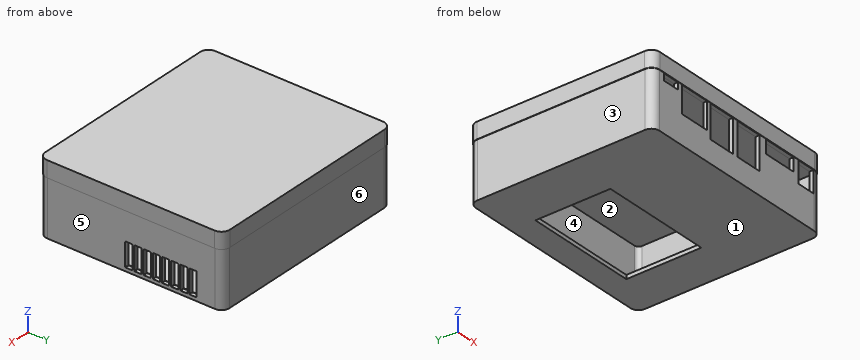
```python
from build123d import *

# Parameters (mm, degrees)
BOSS_EXTRUDE1_DEPTH = 2
BOSS_EXTRUDE2_DEPTH = 8.3
SKETCH3_W           = 57.8
SKETCH3_H           = 38.4
BOSS_EXTRUDE3_DEPTH = 2
BOSS_EXTRUDE6_DEPTH = 30
SKETCH5_W           = 9.3
SKETCH5_H           = 11
SKETCH5_W_2         = 17.696
SKETCH5_H_2         = 6.81
SKETCH5_W_3         = 14.05
SKETCH5_H_3         = 16.84
SKETCH5_W_4         = 8.89
SKETCH5_H_4         = 3.43
SKETCH5_W_5         = 8.74
SKETCH5_H_5         = 13.649992795
SKETCH5_W_6         = 2
SKETCH5_W_7         = 1.707
CUT_EXTRUDE1_DEPTH  = 2
CUT_EXTRUDE2_DEPTH  = 2
CUT_EXTRUDE3_DEPTH  = 2
CUT_EXTRUDE4_DEPTH  = 2


with BuildPart() as part:
    # Sketch1 → Boss-Extrude1 (new body)
    with BuildSketch(Plane.XY):
        with BuildLine():
            Line((-86.3, 47.45), (-86.3, -38.45))
            ThreePointArc((-86.3, -38.45), (-85.626345597, -40.076345597), (-84, -40.75))
            Line((-84, -40.75), (14.4, -40.75))
            ThreePointArc((14.4, -40.75), (16.026345597, -40.076345597), (16.7, -38.45))
            Line((16.7, -38.45), (16.7, 47.45))
            ThreePointArc((16.7, 47.45), (16.026345597, 49.076345597), (14.4, 49.75))
            Line((14.4, 49.75), (-84, 49.75))
            ThreePointArc((-84, 49.75), (-85.626345597, 49.076345597), (-86.3, 47.45))
        make_face()
    extrude(amount=BOSS_EXTRUDE1_DEPTH)

    # Sketch2 → Boss-Extrude2 (add)
    with BuildSketch(Plane.XY.offset(2)):
        with BuildLine():
            Line((-88.3, 47.45), (-88.3, -38.45))
            ThreePointArc((-88.3, -38.45), (-87.040559159, -41.490559159), (-84, -42.75))
            Line((-84, -42.75), (14.4, -42.75))
            ThreePointArc((14.4, -42.75), (17.440559159, -41.490559159), (18.7, -38.45))
            Line((18.7, -38.45), (18.7, 47.45))
            ThreePointArc((18.7, 47.45), (17.440559159, 50.490559159), (14.4, 51.75))
            Line((14.4, 51.75), (-84, 51.75))
            ThreePointArc((-84, 51.75), (-87.040559159, 50.490559159), (-88.3, 47.45))
        make_face()
    extrude(amount=-BOSS_EXTRUDE2_DEPTH)



with BuildPart() as body_2:
    # Sketch3 → Boss-Extrude3 (new body)
    with BuildSketch(Plane(origin=(0, 0, -34.766), x_dir=(-1, 0, 0), z_dir=(0, 0, -1))):
        with BuildLine():
            Line((-14.4, -40.55), (84, -40.55))
            ThreePointArc((84, -40.55), (85.48492424, -39.93492424), (86.1, -38.45))
            Line((86.1, -38.45), (86.1, 47.45))
            ThreePointArc((86.1, 47.45), (85.48492424, 48.93492424), (84, 49.55))
            Line((84, 49.55), (-14.4, 49.55))
            ThreePointArc((-14.4, 49.55), (-15.88492424, 48.93492424), (-16.5, 47.45))
            Line((-16.5, 47.45), (-16.5, -38.45))
            ThreePointArc((-16.5, -38.45), (-15.88492424, -39.93492424), (-14.4, -40.55))
        make_face()
        with Locations((32.8, 19.76)):
            Rectangle(SKETCH3_W, SKETCH3_H, mode=Mode.SUBTRACT)
    extrude(amount=-BOSS_EXTRUDE3_DEPTH)


with BuildPart() as part_1:
    add(part.part)

    add(body_2.part)  # Boss-Extrude6 merges body 2
    # Sketch4 → Boss-Extrude6 (add)
    with BuildSketch(Plane(origin=(0, 0, -34.766), x_dir=(-1, 0, 0), z_dir=(0, 0, -1))):
        with BuildLine():
            Line((84, 51.55), (-14.4, 51.55))
            ThreePointArc((-14.4, 51.55), (-17.299137803, 50.349137803), (-18.5, 47.45))
            Line((-18.5, 47.45), (-18.5, -38.45))
            ThreePointArc((-18.5, -38.45), (-17.299137803, -41.349137803), (-14.4, -42.55))
            Line((-14.4, -42.55), (84, -42.55))
            ThreePointArc((84, -42.55), (86.899137803, -41.349137803), (88.1, -38.45))
            Line((88.1, -38.45), (88.1, 47.45))
            ThreePointArc((88.1, 47.45), (86.899137803, 50.349137803), (84, 51.55))
        make_face()
        with BuildLine():
            ThreePointArc((-16.5, -38.45), (-15.88492424, -39.93492424), (-14.4, -40.55))
            Line((-14.4, -40.55), (84, -40.55))
            ThreePointArc((84, -40.55), (85.48492424, -39.93492424), (86.1, -38.45))
            Line((86.1, -38.45), (86.1, 47.45))
            ThreePointArc((86.1, 47.45), (85.48492424, 48.93492424), (84, 49.55))
            Line((84, 49.55), (-14.4, 49.55))
            ThreePointArc((-14.4, 49.55), (-15.88492424, 48.93492424), (-16.5, 47.45))
            Line((-16.5, 47.45), (-16.5, -38.45))
        make_face(mode=Mode.SUBTRACT)
    extrude(amount=-BOSS_EXTRUDE6_DEPTH)

    # Sketch5 → Cut-Extrude1 (cut)
    with BuildSketch(Plane.XZ.offset(42.55)):
        with Locations((9.2, -11.97)):
            Rectangle(SKETCH5_W, SKETCH5_H)
        with Locations((-7.56, -9.9512)):
            Rectangle(SKETCH5_W_2, SKETCH5_H_2)
        with Locations((-27.4, -14.9662)):
            Rectangle(SKETCH5_W_3, SKETCH5_H_3)
        with Locations((-44.4, -14.9662)):
            Rectangle(SKETCH5_W_3, SKETCH5_H_3)
        with Locations((-76.775, -8.2612)):
            Rectangle(SKETCH5_W_4, SKETCH5_H_4)
        with Locations((-61.75, -13.294996398)):
            Rectangle(SKETCH5_W_5, SKETCH5_H_5)
        with Locations((-56.38, -13.294996398)):
            Rectangle(SKETCH5_W_6, SKETCH5_H_5)
        with Locations((-67.12, -13.294996398)):
            Rectangle(SKETCH5_W_6, SKETCH5_H_5)
        with Locations((-54.5265, -13.294996398)):
            Rectangle(SKETCH5_W_7, SKETCH5_H_5)
        with Locations((-68.9735, -13.294996398)):
            Rectangle(SKETCH5_W_7, SKETCH5_H_5)
    extrude(amount=-CUT_EXTRUDE1_DEPTH, mode=Mode.SUBTRACT)

    # Sketch6 → Cut-Extrude2 (cut)
    with BuildSketch(Plane(origin=(18.5, 0, 0), x_dir=(0, 0, -1), z_dir=(1, 0, 0))):
        with BuildLine():
            Line((32.966, 1.76), (32.966, 4.86))
            ThreePointArc((32.966, 4.86), (32.878132034, 5.072132034), (32.666, 5.16))
            Line((32.666, 5.16), (21.066, 5.16))
            ThreePointArc((21.066, 5.16), (20.853867966, 5.072132034), (20.766, 4.86))
            Line((20.766, 4.86), (20.766, 1.76))
            ThreePointArc((20.766, 1.76), (20.853867966, 1.547867966), (21.066, 1.46))
            Line((21.066, 1.46), (32.666, 1.46))
            ThreePointArc((32.666, 1.46), (32.878132034, 1.547867966), (32.966, 1.76))
        make_face()
    extrude(amount=-CUT_EXTRUDE2_DEPTH, mode=Mode.SUBTRACT)

    # Sketch7 → Cut-Extrude3 (cut)
    with BuildSketch(Plane(origin=(18.5, 0, 0), x_dir=(0, 0, -1), z_dir=(1, 0, 0))):
        with BuildLine():
            Line((20.766, 28.36), (20.766, 25.26))
            ThreePointArc((20.766, 25.26), (20.853867966, 25.047867966), (21.066, 24.96))
            Line((21.066, 24.96), (32.666, 24.96))
            ThreePointArc((32.666, 24.96), (32.878132034, 25.047867966), (32.966, 25.26))
            Line((32.966, 25.26), (32.966, 28.36))
            ThreePointArc((32.966, 28.36), (32.878132034, 28.572132034), (32.666, 28.66))
            Line((32.666, 28.66), (21.066, 28.66))
            ThreePointArc((21.066, 28.66), (20.853867966, 28.572132034), (20.766, 28.36))
        make_face()
        with BuildLine():
            Line((32.666, 23.96), (21.066, 23.96))
            ThreePointArc((21.066, 23.96), (20.853867966, 23.872132034), (20.766, 23.66))
            Line((20.766, 23.66), (20.766, 20.56))
            ThreePointArc((20.766, 20.56), (20.853867966, 20.347867966), (21.066, 20.26))
            Line((21.066, 20.26), (32.666, 20.26))
            ThreePointArc((32.666, 20.26), (32.878132034, 20.347867966), (32.966, 20.56))
            Line((32.966, 20.56), (32.966, 23.66))
            ThreePointArc((32.966, 23.66), (32.878132034, 23.872132034), (32.666, 23.96))
        make_face()
        with BuildLine():
            Line((32.666, 15.56), (21.066, 15.56))
            ThreePointArc((21.066, 15.56), (20.853867966, 15.647867966), (20.766, 15.86))
            Line((20.766, 15.86), (20.766, 18.96))
            ThreePointArc((20.766, 18.96), (20.853867966, 19.172132034), (21.066, 19.26))
            Line((21.066, 19.26), (32.666, 19.26))
            ThreePointArc((32.666, 19.26), (32.878132034, 19.172132034), (32.966, 18.96))
            Line((32.966, 18.96), (32.966, 15.86))
            ThreePointArc((32.966, 15.86), (32.878132034, 15.647867966), (32.666, 15.56))
        make_face()
        with BuildLine():
            Line((32.666, 14.56), (21.066, 14.56))
            ThreePointArc((21.066, 14.56), (20.853867966, 14.472132034), (20.766, 14.26))
            Line((20.766, 14.26), (20.766, 11.16))
            ThreePointArc((20.766, 11.16), (20.853867966, 10.947867966), (21.066, 10.86))
            Line((21.066, 10.86), (32.666, 10.86))
            ThreePointArc((32.666, 10.86), (32.878132034, 10.947867966), (32.966, 11.16))
            Line((32.966, 11.16), (32.966, 14.26))
            ThreePointArc((32.966, 14.26), (32.878132034, 14.472132034), (32.666, 14.56))
        make_face()
        with BuildLine():
            Line((20.766, 9.56), (20.766, 6.46))
            ThreePointArc((20.766, 6.46), (20.853867966, 6.247867966), (21.066, 6.16))
            Line((21.066, 6.16), (32.666, 6.16))
            ThreePointArc((32.666, 6.16), (32.878132034, 6.247867966), (32.966, 6.46))
            Line((32.966, 6.46), (32.966, 9.56))
            ThreePointArc((32.966, 9.56), (32.878132034, 9.772132034), (32.666, 9.86))
            Line((32.666, 9.86), (21.066, 9.86))
            ThreePointArc((21.066, 9.86), (20.853867966, 9.772132034), (20.766, 9.56))
        make_face()
    extrude(amount=-CUT_EXTRUDE3_DEPTH, mode=Mode.SUBTRACT)

    # Sketch10 → Cut-Extrude4 (cut)
    with BuildSketch(Plane(origin=(18.5, 0, 0), x_dir=(0, 0, -1), z_dir=(1, 0, 0))):
        with BuildLine():
            Line((32.966, 34.66), (32.966, 37.76))
            ThreePointArc((32.966, 37.76), (32.878132034, 37.972132034), (32.666, 38.06))
            Line((32.666, 38.06), (21.066, 38.06))
            ThreePointArc((21.066, 38.06), (20.853867966, 37.972132034), (20.766, 37.76))
            Line((20.766, 37.76), (20.766, 34.66))
            ThreePointArc((20.766, 34.66), (20.853867966, 34.447867966), (21.066, 34.36))
            Line((21.066, 34.36), (32.666, 34.36))
            ThreePointArc((32.666, 34.36), (32.878132034, 34.447867966), (32.966, 34.66))
        make_face()
        with BuildLine():
            Line((20.766, 33.06), (20.766, 29.96))
            ThreePointArc((20.766, 29.96), (20.853867966, 29.747867966), (21.066, 29.66))
            Line((21.066, 29.66), (32.666, 29.66))
            ThreePointArc((32.666, 29.66), (32.878132034, 29.747867966), (32.966, 29.96))
            Line((32.966, 29.96), (32.966, 33.06))
            ThreePointArc((32.966, 33.06), (32.878132034, 33.272132034), (32.666, 33.36))
            Line((32.666, 33.36), (21.066, 33.36))
            ThreePointArc((21.066, 33.36), (20.853867966, 33.272132034), (20.766, 33.06))
        make_face()
    extrude(amount=-CUT_EXTRUDE4_DEPTH, mode=Mode.SUBTRACT)


solid = part_1.part
```
Check sheet for the modelled part. Datum: model origin and axes. Units: mm. Face numbers are marked on the shaded views. A direction names the side the tool comes from. Give positions to 0.01 mm unless a question says otherwise; leave off trailing zeros. Write each loop counter-clockwise with the first axis right and the second up, starting at its lowest first coordinate (ties: lowest second). Pieces come first, ordered by that corner, then holes.
Item 1: Cross-section at C-C (z = -15). Count the separate pieces of the cut face and the enclosed holes in it, and give its area (3 significant figures).
Item 2: Cross-section at B-B (y = 12.5). Enter the section's corners in (x, z).
Item 3: Access from +Z, -Z, +X, -X, +Y, -Y to the whole of each face (thin tool, end or side, straight path). Record for the marked faces 4, 5 and 6.
Item 4: Draft check along Z on the marked faces 1, 2 and 3. Enter one of: released by +Z, released by -Z, zero draft, split by the parting line, or undercut.
Item 5: Cross-section at D-D (y = -11). Enter the section's corners in (x, z), and give its area (3 significant figures).
Item 6: Cross-section at A-A (x = -10). Enter the section's corners in (y, z), and give its area (3 significant figures).
Item 7: Gauge pin test, flat ends, axial feed: pin 1 (3 mm diameter, centred on y = -10.5, z = -18.5, fed in from -X); pin 2 (8.5 mm diameter, centred on y = 17.5, z = -21.5, fed in from +X); pin 3 (2 mm diameter, centred on y = -41.5, z = -9.5, fed in from +X). Record the tip position at first contact, or that the pin passes through.
Item 8: Scan lines: L1, parallel to Z at x = -68, y = 2; L2, parallel to Y at x = -66, z = -27; L3, parallel to X at y = -18.5, z = -7.5. Record each from-to range of solid material in increasing order.
Report:
1. separate pieces: 4
1. enclosed holes: 0
1. area: 669 mm2
2. outline: (-88.3, -6.3) - (-88.1, -6.3) - (-88.1, -34.77) - (-61.7, -34.77) - (-61.7, -32.77) - (-86.1, -32.77) - (-86.1, -6.3) - (16.5, -6.3) - (16.5, -20.77) - (18.5, -20.77) - (18.5, -6.3) - (18.7, -6.3) - (18.7, 2) - (-88.3, 2) - close; (-3.9, -34.77) - (18.5, -34.77) - (18.5, -32.97) - (16.5, -32.97) - (16.5, -32.77) - (-3.9, -32.77) - close
3. face 4: none
3. face 5: -Z, +X, +Y, -Y
3. face 6: -Z, +X, -X, +Y
4. face 1: released by -Z
4. face 2: undercut
4. face 3: zero draft
5. outline: (-88.3, -6.3) - (-88.1, -6.3) - (-88.1, -34.77) - (18.5, -34.77) - (18.5, -6.3) - (18.7, -6.3) - (18.7, 2) - (-88.3, 2) - close; hole (-86.1, -32.77) - (16.5, -32.77) - (16.5, -6.3) - (-86.1, -6.3) - close
5. area: 1,210 mm2
6. outline: (-42.75, -6.3) - (-42.55, -6.3) - (-42.55, -6.55) - (-40.55, -6.55) - (-40.55, -6.3) - (49.55, -6.3) - (49.55, -32.77) - (38.96, -32.77) - (38.96, -34.77) - (51.55, -34.77) - (51.55, -6.3) - (51.75, -6.3) - (51.75, 2) - (-42.75, 2) - close; (-42.55, -34.77) - (0.56, -34.77) - (0.56, -32.77) - (-40.55, -32.77) - (-40.55, -13.36) - (-42.55, -13.36) - close
6. area: 988 mm2
7. pin 1: stops at x = -88.1
7. pin 2: stops at x = 18.5
7. pin 3: stops at x = 17.95
8. L1: z = -34.77 to -32.77, -6.3 to 2
8. L2: y = -42.55 to -40.55, 49.55 to 51.55
8. L3: x = -88.1 to -86.1, 16.5 to 18.5
